Could you check a few things on this drawing? It's one solid part, dimensions in mm from its lowest x, y, z. A direction names the side the tool comes from. Give positions to 0.01 mm unless a question says otherwise; leave off trailing zeros. Write each loop counter-clockwise with the first axis right and the second up, starting at its lowest first coordinate (ties: lowest second). Pieces come first, ordered by that corner, then holes. Notation, with made-up numbers: (4, 4) - (54, 4) arc R22 ccw to (54, 29) - close; hole circle Ø9 at (13.5, 9). An arc over 180 degrees is marked (long way). One line per item, written item: value. Start each with the question number.
1) I'm going to push a flat-ended pin straight in: P1, Ø1.6, axis at y = 3.5, z = 2.5, coming from the -X side. Where does the tip first touch, or does it pass through?
2) Imagine slicing it at B-B on z = 2.95. Write out the boundary of the cut face in (x, y).
3) Imagine slicing it at A-A on y = 4.15. Write out the boundary of the cut face in (x, z), plus the area to 3 significant figures.
4) On a 3-axis mill with a long thin cutter (end or side, diameter ignored), from which of +Z, -Z, +X, -X, +Y, -Y can I reach the whole of each face in a straight line? I mean the marked faces 1 and 2. Say none if no direction works.
5) Imagine slicing it at D-D on y = 4.9. Write out the boundary of the cut face in (x, z).
6) Imagine slicing it at C-C on x = 4.5. Write out the boundary of the cut face in (y, z).
7) Please list where these lines run through material, in increasing order: L1, parallel to X at y = 1.5, z = 1.8; L2, parallel to Z at x = 4.25, y = 5.25; L3, parallel to Y at x = 4, z = 3.7. Write a range as [from, to].
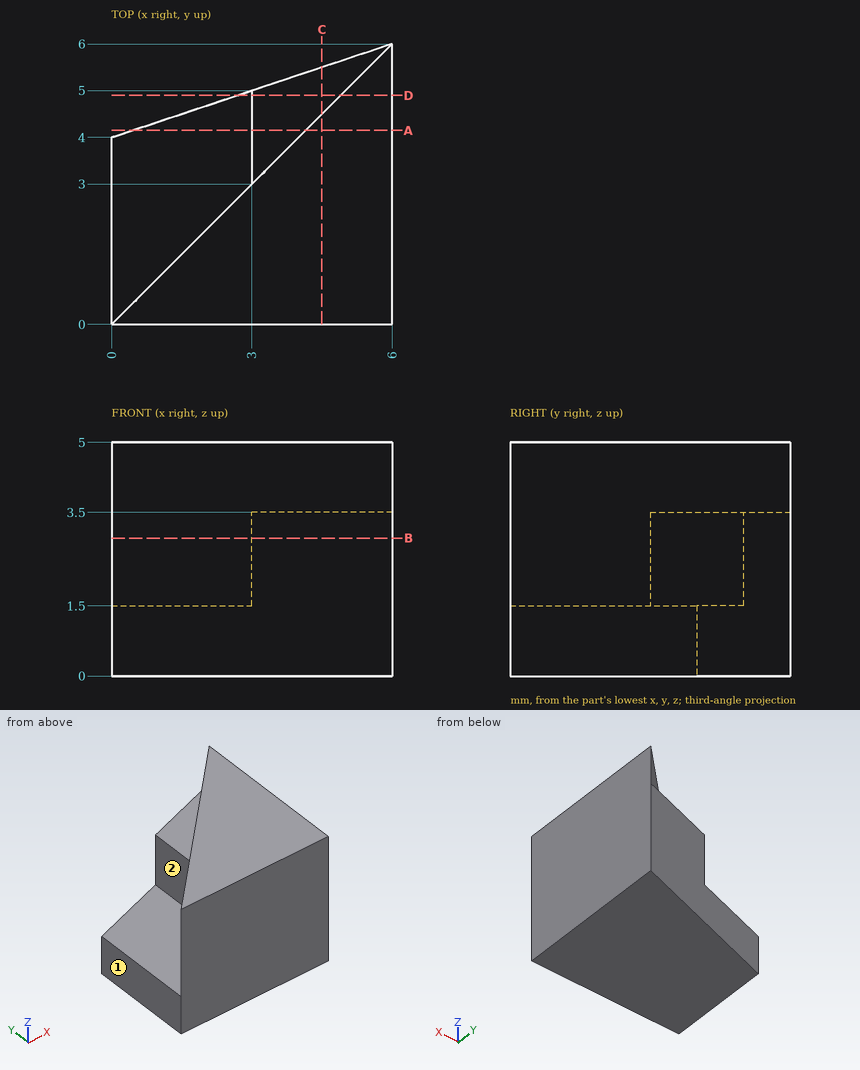
Numbers:
1. P1: x = 2.7
2. outline: (0, 0) - (6, 0) - (6, 6) - (3, 5) - (3, 3) - close
3. outline: (0.45, 0) - (6, 0) - (6, 5) - (4.15, 5) - (4.15, 3.5) - (3, 3.5) - (3, 1.5) - (0.45, 1.5) - close
3. area: 17.1 mm^2
4. face 1: +Z, -Z, -X, +Y, -Y
4. face 2: +Z, -X, +Y
5. outline: (2.7, 0) - (6, 0) - (6, 5) - (4.9, 5) - (4.9, 3.5) - (3, 3.5) - (3, 1.5) - (2.7, 1.5) - close
6. outline: (0, 0) - (5.5, 0) - (5.5, 3.5) - (4.5, 3.5) - (4.5, 5) - (0, 5) - close
7. L1: [1.5, 6]
7. L2: [0, 3.5]
7. L3: [0, 4]
